```python
from build123d import *

# Parameters (mm, degrees)
SKETCH_1_W      = 21
SKETCH_1_H      = 25
SKETCH_1_R      = 1.05
EXTRUDE_1_DEPTH = 2
SKETCH_2_W      = 9
SKETCH_2_H      = 1.1
EXTRUDE_2_DEPTH = 0.72
FILLET_1_R      = 2
FILLET_3_R      = 0.4


with BuildPart() as part:
    # 草图1 → 凸台-拉伸1 (new body)
    with BuildSketch(Plane.XY):
        with Locations((10.5, -12.5)):
            Rectangle(SKETCH_1_W, SKETCH_1_H)
        with Locations((3, -5)):
            Circle(SKETCH_1_R, mode=Mode.SUBTRACT)
        with Locations((18, -5)):
            Circle(SKETCH_1_R, mode=Mode.SUBTRACT)
        with Locations((3, -20)):
            Circle(SKETCH_1_R, mode=Mode.SUBTRACT)
        with Locations((18, -20)):
            Circle(SKETCH_1_R, mode=Mode.SUBTRACT)
    extrude(amount=EXTRUDE_1_DEPTH)

    # 草图2 → 凸台-拉伸2 (add)
    with BuildSketch(Plane.XY.offset(2)):
        with Locations((10.5, -5.05)):
            Rectangle(SKETCH_2_W, SKETCH_2_H)
        with Locations((10.5, -8.05)):
            Rectangle(SKETCH_2_W, SKETCH_2_H)
        with Locations((10.5, -11.05)):
            Rectangle(SKETCH_2_W, SKETCH_2_H)
        with Locations((10.5, -14.05)):
            Rectangle(SKETCH_2_W, SKETCH_2_H)
        with Locations((10.5, -17.05)):
            Rectangle(SKETCH_2_W, SKETCH_2_H)
        with Locations((10.5, -20.05)):
            Rectangle(SKETCH_2_W, SKETCH_2_H)
    extrude(amount=EXTRUDE_2_DEPTH)

    # 圆角1
    fillet_1_edges = [part.edges().sort_by_distance(p)[0] for p in [
        (0, 0, 1),
        (21, 0, 1),
        (21, -25, 1),
        (0, -25, 1),
    ]]
    fillet(fillet_1_edges, radius=FILLET_1_R)

    # 圆角3
    fillet_3_edges = [part.edges().sort_by_distance(p)[0] for p in [
        (10.5, -5.6, 2.72),
        (10.5, -4.5, 2.72),
        (10.5, -7.5, 2.72),
        (10.5, -8.6, 2.72),
        (10.5, -10.5, 2.72),
        (10.5, -11.6, 2.72),
        (10.5, -13.5, 2.72),
        (10.5, -14.6, 2.72),
        (10.5, -16.5, 2.72),
        (10.5, -17.6, 2.72),
        (10.5, -19.5, 2.72),
        (10.5, -20.6, 2.72),
    ]]
    fillet(fillet_3_edges, radius=FILLET_3_R)


solid = part.part
```
Geometry: final body of the model. Coordinates: model frame, mm. Round coordinates to 2 decimals unless told otherwise and drop trailing zeros. Loops run counter-clockwise (first coordinate to the right, second up) from the corner with the lowest first, then second, coordinate; pieces in that order, holes last. Notation, with made-up numbers: (87.5, 36) -> (137.5, 36) arc R21 ccw to (137.5, 72) -> close; hole circle Ø11 at (63, -32.5). An arc over 180 degrees is marked (long way). Use one line per item in the form item = value. Start each with the question number.
1) Section B-B on z = 1.6. Output: boundary loops of the cut face in (x, y).
2) Draft query along Y for faces 1 (the cylindrical face through (0.57, -0.6, 1.01)), 2 (the flat face through (21, -13, 1)), 3 (the flat face through (10, -12, 2)), 4 (the flat face through (10, -25, 1)). Return one class per face: released by +Y, released by -Y, zero draft, split by the parting line, or undercut.
3) Section C-C on x = 18.5. Output: boundary loops of the cut face in (y, z), then the cut area to 3 significant figures.
4) Line query: L1, parallel to Y at x = 18, z = 0.8; L2, parallel to Z at x = 14, y = -21.5; L3, parallel to Y at x = 10.5, z = 2.5. Output: solid intervals per line, ascending.
5) Section A-A on x = 3. Output: boundary loops of the cut face in (y, z), then the cut area to 3 significant figures.
6) Section D-D on x = 16. Output: boundary loops of the cut face in (y, z), then the cut area to 3 significant figures.
7) First-contact query: P1, Ø3.5, axis at x = 18, y = -20, coming from the +Z side; P2, Ø5, axis at x = 8, y = -17, coming from the -Z side; P3, Ø0.8, axis at y = -11, z = 2.5, coming from the +X side. Flat tips, straight axial feed; report the tip coordinate or a pass-through.
Response:
q1.outline = (0, -23) arc R2 ccw to (2, -25) -> (19, -25) arc R2 ccw to (21, -23) -> (21, -2) arc R2 ccw to (19, 0) -> (2, 0) arc R2 ccw to (0, -2) -> close; hole circle Ø2.1 at (3, -20); hole circle Ø2.1 at (3, -5); hole circle Ø2.1 at (18, -20); hole circle Ø2.1 at (18, -5)
q2.face_1 = released by +Y
q2.face_2 = zero draft
q2.face_3 = undercut
q2.face_4 = released by -Y
q3.outline = (-25, 0) -> (-20.92, 0) -> (-20.92, 2) -> (-25, 2) -> close; (-19.08, 0) -> (-5.92, 0) -> (-5.92, 2) -> (-19.08, 2) -> close; (-4.08, 0) -> (0, 0) -> (0, 2) -> (-4.08, 2) -> close
q3.area = 42.6 mm^2
q4.L1 = -25 to -21.05, -18.95 to -6.05, -3.95 to 0
q4.L2 = 0 to 2
q4.L3 = -20.56 to -19.54, -17.56 to -16.54, -14.56 to -13.54, -11.56 to -10.54, -8.56 to -7.54, -5.56 to -4.54
q5.outline = (-25, 0) -> (-21.05, 0) -> (-21.05, 2) -> (-25, 2) -> close; (-18.95, 0) -> (-6.05, 0) -> (-6.05, 2) -> (-18.95, 2) -> close; (-3.95, 0) -> (0, 0) -> (0, 2) -> (-3.95, 2) -> close
q5.area = 41.6 mm^2
q6.outline = (-25, 0) -> (0, 0) -> (0, 2) -> (-25, 2) -> close
q6.area = 50.0 mm^2
q7.P1 = 2
q7.P2 = 0
q7.P3 = 15
